Read the model definition and answer for the solid it produces. Units are mm, in the model's axes. Coordinates: 2 decimals unless noted, no trailing zeros. Order: outer loops, then holes, each group sorted by start corner. A loop starts at its lowest first (then second) coordinate and runs counter-clockwise, first axis right, second up. Notation, with made-up numbers: (33, 42.25) -> (49, 42.25) arc R23 cw to (49, 59.25) -> close; hole circle Ø8 at (70.5, -18). An arc over 180 degrees is marked (long way). Return JSON: item names as keys, results as strings. Group by question number.
```python
from build123d import *

# Parameters (mm, degrees)
F1_DEPTH = 10.0076
F2_W     = 50.8
F2_H     = 25.4
F3_DEPTH = 10.0086
F4_R     = 76.2
F5_DEPTH = 10.0086


with BuildPart() as f1:
    # F0 (on Front) → F1 (new body)
    with BuildSketch(Plane.XZ):
        Polygon((711.428056, 899.191029), (-507.771944, 899.191029), (-507.771944, -1056.608971), (317.728056, -1056.608971), (317.728056, -320.008971), (711.428056, -320.008971), align=None)
    extrude(amount=F1_DEPTH)

    # F2 (on face) → F3 (cut, through all)
    with BuildSketch(Plane.XZ.offset(10.0076)):
        with Locations((686.028056, 886.491029)):
            Rectangle(F2_W, F2_H)
        with Locations((-482.371944, 886.491029)):
            Rectangle(F2_W, F2_H)
        with Locations((686.028056, -307.308971)):
            Rectangle(F2_W, F2_H)
        with Locations((-482.371944, -307.308971)):
            Rectangle(F2_W, F2_H)
        with Locations((-12.471944, -307.308971)):
            Rectangle(F2_W, F2_H)
    extrude(amount=-F3_DEPTH, mode=Mode.SUBTRACT)

    # F4 (on face) → F5 (cut, through all)
    with BuildSketch(Plane.XZ.offset(10.0076)):
        with Locations((-101.371944, 594.391029)):
            Circle(F4_R)
    extrude(amount=-F5_DEPTH, mode=Mode.SUBTRACT)


solid = f1.part
```
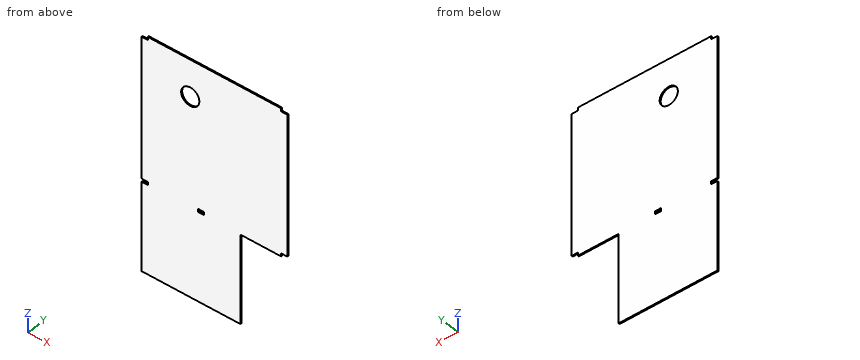
1. Straight lines are drawn through the part: L1, parallel to Z at x = 523.5, y = -5.25; L2, parallel to X at y = -5.75, z = -610; L3, parallel to X at y = -8.5, z = 624. For each, find the intervals that lie inside material, in ascending order.
2. Find section A-A on y = -6.25. Determine the outline of the cut face in (x, z), and give its area (3 significant figures).
3. Find section B-B on x = 433.5. Determine the outline of the cut face in (y, z).
4. Find section C-C on z = -676. Determine the outline of the cut face in (x, y).
5. Given pin 1 (3 mm diameter, centred on y = -3, z = -303.5, fed in from -X); pin 2 (2 mm diameter, centred on x = 450, y = -3.5, fed in from -Z); pin 3 (5 mm diameter, centred on y = -6, z = 888.5, fed in from +X); pin 4 (1.5 mm diameter, centred on x = -76.5, z = -663.5, fed in from +Y), each flat-ended and moving along its own axis, determine where each tip first touches the part or whether it passes through.
Result:
{
 "1": {"L1": "-320.01 to 899.19", "L2": "-507.77 to 317.73", "L3": "-507.77 to -171.58, -31.16 to 711.43"},
 "2": {"outline": "(-507.77, -1056.61) -> (317.73, -1056.61) -> (317.73, -320.01) -> (660.63, -320.01) -> (660.63, -294.61) -> (711.43, -294.61) -> (711.43, 873.79) -> (660.63, 873.79) -> (660.63, 899.19) -> (-456.97, 899.19) -> (-456.97, 873.79) -> (-507.77, 873.79) -> (-507.77, -294.61) -> (-456.97, -294.61) -> (-456.97, -320.01) -> (-507.77, -320.01) -> close; hole circle Ø152.4 at (-101.37, 594.39); hole (-37.87, -320.01) -> (12.93, -320.01) -> (12.93, -294.61) -> (-37.87, -294.61) -> close", "area": "2,070,000 mm^2"},
 "3": {"outline": "(-10.01, -320.01) -> (0, -320.01) -> (0, 899.19) -> (-10.01, 899.19) -> close"},
 "4": {"outline": "(-507.77, -10.01) -> (317.73, -10.01) -> (317.73, 0) -> (-507.77, 0) -> close"},
 "5": {"pin 1": "x = -456.97", "pin 2": "z = -320.01", "pin 3": "x = 660.63", "pin 4": "y = 0"}
}
